Geometry: final body of the model. Coordinates: model frame, mm. Round coordinates to 2 decimals unless told otherwise and drop trailing zeros. Loops run counter-clockwise (first coordinate to the right, second up) from the corner with the lowest first, then second, coordinate; pieces in that order, holes last. Notation, with made-up numbers: (-7.75, 64) - (51.25, 64) arc R33 cw to (51.25, 95) - close; hole circle Ø2 at (79, 76). An arc over 180 degrees is marked (long way). Return JSON: item names as keys, results as strings. Group by question number.
1. Section B-B on y = -7. Return loops of the section in (x, z).
2. Draft query along Y for faces 1 (the face through (29.716, -18.885, 1.479)), 2 (the face through (-1, -28, 1)), 3 (the face through (-1, 0, 0)). Return one class per face: +Y half, -Y half, draft (parallel to the pull), parting line (faces both ways), or undercut.
3. Section A-A on z = 2.35. Count the separate pieces of the cut face and the enclosed holes in it, and give its area (3 significant figures).
4. Material intervals for probe 1 along X at (y, z) = (-21, 0.75); probe 2 along X at (y, z) = (-20.5, 2.6); probe 3 along Y at (x, z) = (-29, 2), sorted ascending.
from build123d import *

# Parameters (mm, degrees)
SKETCH_1_W          = 75
SKETCH_1_H          = 56
EXTRUDE_1_DEPTH     = 3
SKETCH_2_R          = 1.65
CUT_EXTRUDE_1_DEPTH = 3
SKETCH_4_R          = 1.65
CUT_EXTRUDE_3_DEPTH = 8


with BuildPart() as part:
    # 草图1 → 凸台-拉伸1 (new body)
    with BuildSketch(Plane.XY):
        Rectangle(SKETCH_1_W, SKETCH_1_H)
    extrude(amount=EXTRUDE_1_DEPTH)

    # 草图2 → 切除-拉伸1 (cut)
    with BuildSketch(Plane(origin=(0, 0, 0), x_dir=(-1, 0, 0), z_dir=(0, 0, -1))):
        with Locations((-28.5, 20)):
            Circle(SKETCH_2_R)
        with Locations((28.5, 20)):
            Circle(SKETCH_2_R)
        with Locations((-28.5, -20)):
            Circle(SKETCH_2_R)
        with Locations((28.5, -20)):
            Circle(SKETCH_2_R)
    extrude(amount=-CUT_EXTRUDE_1_DEPTH, mode=Mode.SUBTRACT)

    # 草图4 → 切除-拉伸3 (cut)
    with BuildSketch(Plane(origin=(0, 0, 0), x_dir=(-1, 0, 0), z_dir=(0, 0, -1))):
        with Locations((-29.5, 5)):
            Circle(SKETCH_4_R)
        with Locations((29.5, 5)):
            Circle(SKETCH_4_R)
        with Locations((-29.5, -7)):
            Circle(SKETCH_4_R)
        with Locations((29.5, -7)):
            Circle(SKETCH_4_R)
    extrude(amount=-CUT_EXTRUDE_3_DEPTH, mode=Mode.SUBTRACT)


solid = part.part
Taken from the geometry:
{
 "1": {"outline": "(-37.5, 0) - (-31.15, 0) - (-31.15, 3) - (-37.5, 3) - close; (-27.85, 0) - (27.85, 0) - (27.85, 3) - (-27.85, 3) - close; (31.15, 0) - (37.5, 0) - (37.5, 3) - (31.15, 3) - close"},
 "2": {"face 1": "undercut", "face 2": "-Y half", "face 3": "draft"},
 "3": {"separate pieces": "1", "enclosed holes": "8", "area": "4,130 mm2"},
 "4": {"probe 1": "-37.5 to -29.81, -27.19 to 27.19, 29.81 to 37.5", "probe 2": "-37.5 to -30.07, -26.93 to 26.93, 30.07 to 37.5", "probe 3": "-28 to -21.57, -18.43 to -8.57, -5.43 to 3.43, 6.57 to 18.43, 21.57 to 28"}
}
